Could you check a few things on this model? Use its own coordinates, in mm. Round coordinates to 2 decimals unless told otherwise and drop trailing zeros. Write each loop counter-clockwise with the first axis right and the second up, starting at its lowest first coordinate (ties: lowest second). Pieces come first, ordered by that corner, then holes. Notation, with made-up numbers: M 84,25.25 L 122,25.25 A37 ccw 122,63.25 Z; hole C 9.25,-5 d8. An arc over 180 degrees is marked long. One line per item, written item: value. Start each with the question number.
(1) I want a section at B-B on y = 292. Please give me the cut outline in (x, z), and give its area (3 significant figures).
(2) I want a section at A-A on z = -16.5. Please give me the cut outline in (x, y).
(3) If I drill on L1, parallel to Z at x = 450, y = 276 (3 decimals); L2, parallel to X at y = 272, z = -27; L3, parallel to X at y = 288.5, z = -24, over which ranges is the centre line in solid material (lowest first)?
(4) I'm going to push flat-ended pins straight in: pin 1 Ø10 at (x, y) = (427.5, 246.5) entering from +Z (3 decimals); pin 2 Ø12 at (y, z) = (288, -14.5) entering from -X; pin 3 Ø1.5 at (y, z) = (256.5, -21) entering from -X. Where does each tip first touch, or does it pass through?
```python
from build123d import *

# Parameters (mm, degrees)
BOSS_EXTRUDE1_DEPTH = 31.75
SKETCH3_W           = 3.175
SKETCH3_H           = 19.05
CUT_EXTRUDE1_DEPTH  = 3.175


with BuildPart() as part:
    # Sketch1 → Boss-Extrude1 (new body)
    with BuildSketch(Plane.XY):
        Polygon((423.30572032, 238.067163043), (470.193893436, 314.999977905), (472.905042097, 313.347616582), (426.01686898, 236.41480172), align=None)
    extrude(amount=-BOSS_EXTRUDE1_DEPTH)

    # Sketch3 → Cut-Extrude1 (cut)
    with BuildSketch(Plane(origin=(205.569888368, -125.288494, 0), x_dir=(0, 0, -1), z_dir=(0.85390509, -0.520428763, 0))):
        with Locations((1.5875, 504.157510823)):
            Rectangle(SKETCH3_W, SKETCH3_H)
        with Locations((30.1625, 504.157510823)):
            Rectangle(SKETCH3_W, SKETCH3_H)
        with Locations((1.5875, 433.112234694)):
            Rectangle(SKETCH3_W, SKETCH3_H)
        with Locations((30.1625, 433.112234694)):
            Rectangle(SKETCH3_W, SKETCH3_H)
        with Locations((30.1625, 468.037234694)):
            Rectangle(SKETCH3_W, SKETCH3_H)
        with Locations((1.5875, 468.037234694)):
            Rectangle(SKETCH3_W, SKETCH3_H)
    extrude(amount=-CUT_EXTRUDE1_DEPTH, mode=Mode.SUBTRACT)


solid = part.part
```
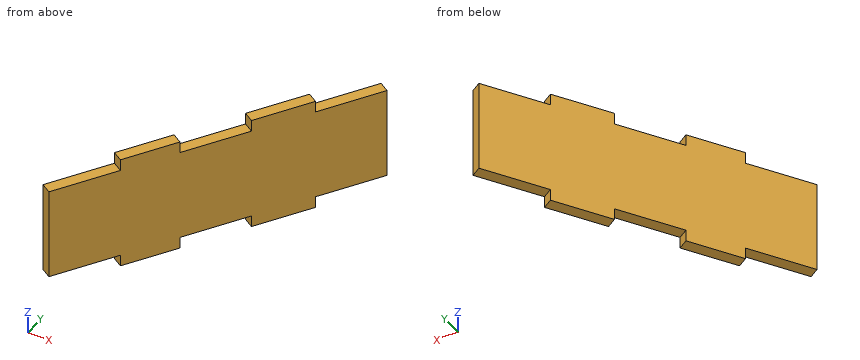
Found:
1. outline: M 456.18,-31.75 L 459.89,-31.75 L 459.89,0 L 456.18,0 Z
1. area: 118 mm²
2. outline: M 423.31,238.07 L 426.02,236.41 L 472.91,313.35 L 470.19,315 Z
3. L1: z = -28.575 to -3.175
3. L2: x = 443.99 to 447.7
3. L3: x = 454.04 to 457.76
4. pin 1: stops at z = -3.175
4. pin 2: stops at x = 450.08
4. pin 3: stops at x = 434.08
